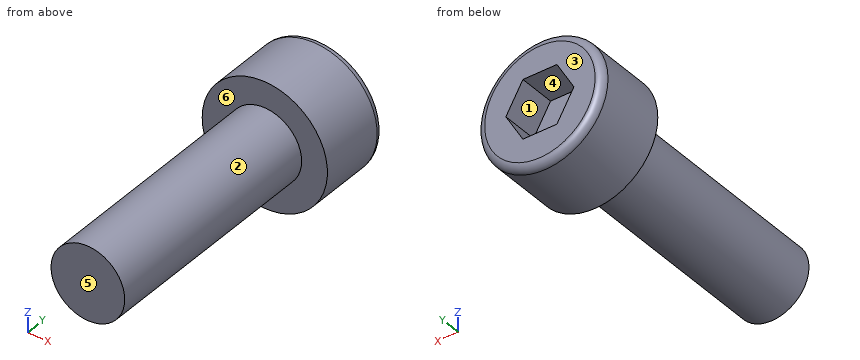
Autodesk Inventor part; units mm, degrees
ref_plane "YZ Plane" through (0, 0, 0) normal (1, 0, 0) x (0, 1, 0)
ref_plane "XZ Plane" through (0, 0, 0) normal (0, 1, 0) x (-1, 0, 0)
ref_plane "XY Plane" through (0, 0, 0) normal (0, 0, 1) x (1, 0, 0)
sketch "Cap Cross Section" plane through (0, 0, 0) normal (0, 1, 0) x (-1, 0, 0)
  circle A0 centre (0, 0) radius 4.25
  dimension "d0" = 8.5
extrude "Cap" add sketch "Cap Cross Section" along normal blind 5
sketch "Key Socket Cutout Outline" plane through (0, 5, 0) normal (0, 1, 0) x (1, 0, 0)
  line L0 (1.1547, 2) -> (2.3094, 0)
  line L1 (2.3094, 0) -> (1.1547, -2)
  line L2 (1.1547, -2) -> (-1.1547, -2)
  line L3 (-1.1547, -2) -> (-2.3094, 0)
  line L4 (-2.3094, 0) -> (-1.1547, 2)
  line L5 (-1.1547, 2) -> (1.1547, 2)
  point P0 (0, 0)
  point P1 (0, 0)
  dimension "d3" = 4
extrude "Key Socket Cutout" cut sketch "Key Socket Cutout Outline" against normal blind 2.5
sketch "Body Cross Section" plane through (0, 0, 0) normal (0, -1, 0) x (1, 0, 0)
  circle A0 centre (0, 0) radius 2.5
  dimension "d6" = 5
extrude "Body" add sketch "Body Cross Section" along normal blind 16
thread "Thread"
fillet "Cap Fillet" radius 0.5 1 edges at (4.25, 5, 0)
properties part number "SSCF-M5-16-A4" material "Stainless Steel AISI 317"
Design review of the part built by this model. Coordinates are the model's own, in mm. Face numbers are marked on the shaded views. A direction names the side the tool comes from. Round coordinates to 2 decimals unless told otherwise and drop trailing zeros. Order: outer loops, then holes, each group sorted by start corner. A loop starts at its lowest first (then second) coordinate and runs counter-clockwise, first axis right, second up. Notation, with made-up numbers: (-20, 11) - (22, 11) arc R10 ccw to (22, 15) - close; hole circle Ø7 at (45, 77.5). An arc over 180 degrees is marked (long way). Return JSON: item names as keys, results as strings.
Q1. Machinability: for the marked faces 5 and 6, which of the approach directions +Z, -Z, +X, -X, +Y, -Y give a long, thin tool a straight path to every point of the face, cutting with its end or side? Answer none if there is none.
Computed values:
{"face 5": "+Z, -Z, +X, -X, -Y", "face 6": "-Y"}
Q2. Consider section A-A on y = 3.5. Write out the cut boundary in (x, z).
Computed values:
{"outline": "circle Ø8.5 at (0, 0); hole (-2.31, 0) - (-1.15, -2) - (1.15, -2) - (2.31, 0) - (1.15, 2) - (-1.15, 2) - close"}
Q3. Wall thickness on L1, parallel to Y at x = -3.25, z = -1.25; L2, parallel to Y at x = -1.25, z = 1.25; L3, parallel to Z at x = -1.5, y = -0.75: over which ranges is each line inside the solid? List them lowest first. Write a range as [from, to].
Computed values:
{"L1": "y = [0, 5]", "L2": "y = [-16, 2.5]", "L3": "z = [-2, 2]"}
Q4. Consider section C-C on y = -3.75. Write out the cut boundary in (x, z), plus the area to 3 significant figures.
Computed values:
{"outline": "circle Ø5 at (0, 0)", "area": "19.6 mm2"}
Q5. For pin 1 Ø4 at (y, z) = (-10.5, 1) entering from +X; pin 2 Ø3 at (y, z) = (-2, -2) entering from +X; pin 3 Ø0.7 at (x, y) = (-0.5, 4) entering from +Z, all flat-tipped, find the tip position at first contact; note any pin that passes through.
Computed values:
{"pin 1": "stops at x = 2.5", "pin 2": "stops at x = 2.45", "pin 3": "stops at z = 4.25"}
Q6. Consider section B-B on x = 0. Write out the cut boundary in (y, z), plus the area to 3 significant figures.
Computed values:
{"outline": "(-16, -2.5) - (0, -2.5) - (0, -4.25) - (4.5, -4.25) arc R0.5 ccw to (5, -3.75) - (5, -2) - (2.5, -2) - (2.5, 2) - (5, 2) - (5, 3.75) arc R0.5 ccw to (4.5, 4.25) - (0, 4.25) - (0, 2.5) - (-16, 2.5) - close", "area": "112 mm2"}
Q7. The part is to be moulded in two halves that separate along Z. For the marked faces 1, 2, 3 and 4, say which applies: pulls with the +Z half, pulls with the -Z half, needs draft (parallel to the pull), parting line crosses it, or undercut.
Computed values:
{"face 1": "undercut", "face 2": "parting line crosses it", "face 3": "needs draft", "face 4": "undercut"}
